Drawing for the job (mm, zero at the part's lowest x, y, z). Round coordinates to 2 decimals unless told otherwise and drop trailing zeros. Order: outer loops, then holes, each group sorted by start corner. A loop starts at its lowest first (then second) coordinate and runs counter-clockwise, first axis right, second up. Notation, with made-up numbers: (46.25, 4.5) -> (60.25, 4.5) arc R29 cw to (60.25, 33.5) -> close; hole circle Ø5 at (37.25, 40.5). An arc over 180 degrees is marked (long way). Answer as CSV lines item,"result". Start each with the question number.
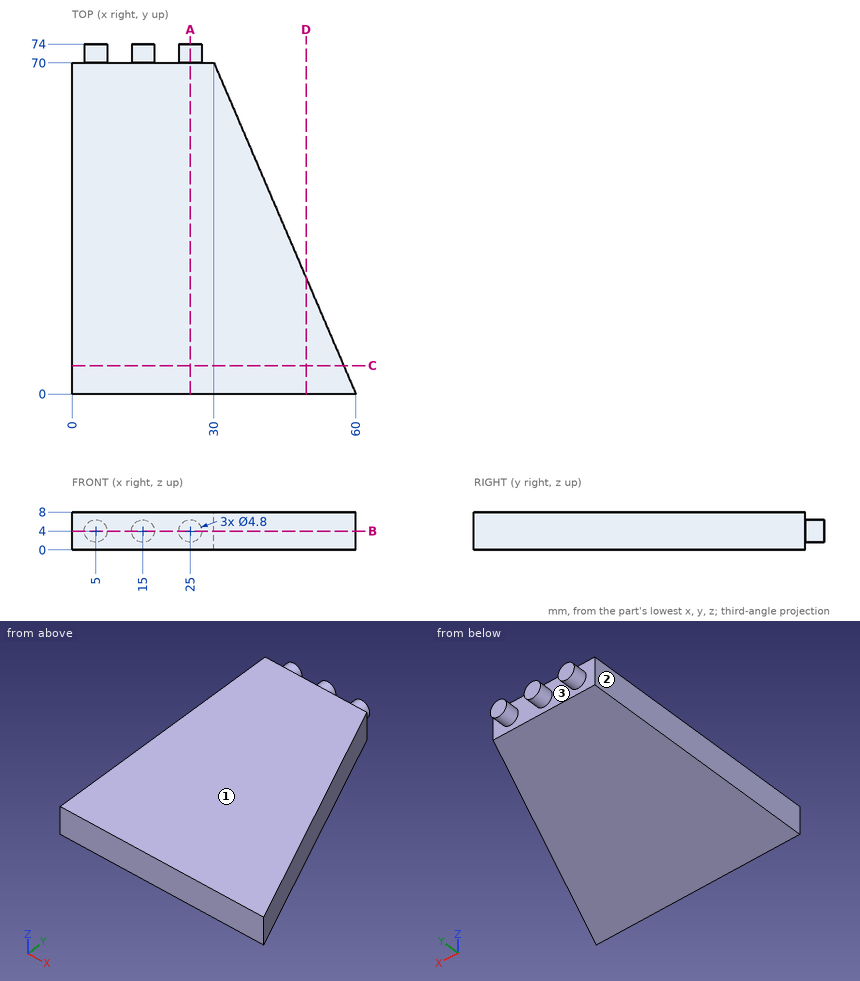
Q1. Slice it at B-B, the plane z = 4. Write the cut outline in (x, y), plus the area to 3 significant figures.
Q2. Slice it at C-C, the plane y = 6. Write the cut outline in (x, z), plus the area to 3 significant figures.
Q3. Slice it at A-A, the plane x = 25. Write the cut outline in (y, z), plus the area to 3 significant figures.
Q4. Probe L1, parallel to Y at x = 29, z = 6.75; L2, parallel to X at y = 26, z = 4.5; L3, parallel to X at y = 55.5, z = 4.25. List the from-to ranges inside material, lowest first.
Q5. Slice it at D-D, the plane x = 49.5. Write the cut outline in (y, z).
Q6. Two-plate mould, pull along X, no slides. Class the marked faces 1, 2 and 3: +X half, -X half, draft (parallel to the pull), parting line (faces both ways), or undercut.
Solutions:
1,outline,"(0, 0) -> (60, 0) -> (30, 70) -> (27.4, 70) -> (27.4, 74) -> (22.6, 74) -> (22.6, 70) -> (17.4, 70) -> (17.4, 74) -> (12.6, 74) -> (12.6, 70) -> (7.4, 70) -> (7.4, 74) -> (2.6, 74) -> (2.6, 70) -> (0, 70) -> close"
1,area,"3,210 mm2"
2,outline,"(0, 0) -> (57.43, 0) -> (57.43, 8) -> (0, 8) -> close"
2,area,"459 mm2"
3,outline,"(0, 0) -> (70, 0) -> (70, 1.6) -> (74, 1.6) -> (74, 6.4) -> (70, 6.4) -> (70, 8) -> (0, 8) -> close"
3,area,"579 mm2"
4,L1,"y = 0 to 70"
4,L2,"x = 0 to 48.86"
4,L3,"x = 0 to 36.21"
5,outline,"(0, 0) -> (24.5, 0) -> (24.5, 8) -> (0, 8) -> close"
6,face 1,"draft"
6,face 2,"-X half"
6,face 3,"undercut"
